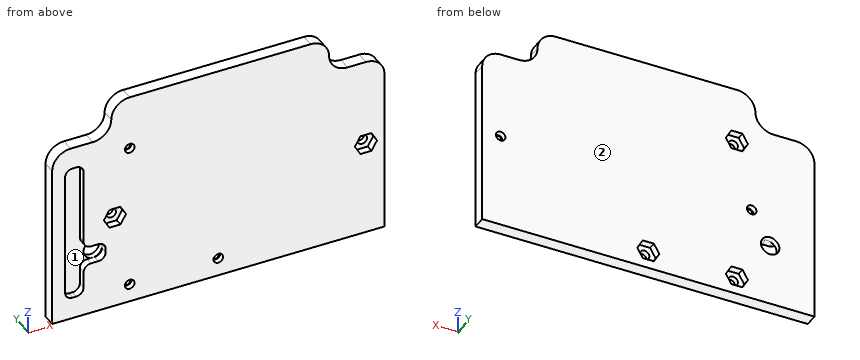
```python
from build123d import *

# Parameters (mm, degrees)
F1_DEPTH  = 4.445
F2_R      = 1.651
F3_DEPTH  = 4.446
F4_R      = 1.651
F5_DEPTH  = 4.446
F7_DEPTH  = 2.54
F9_DEPTH  = 2.54
F10_R     = 3.175
F11_DEPTH = 4.446
F13_DEPTH = 2.54


with BuildPart() as f1:
    # F0 (on Front) → F1 (new body)
    with BuildSketch(Plane.XZ):
        with BuildLine():
            Line((33.804538, 40.817322), (-28.425462, 40.817322))
            ThreePointArc((-28.425462, 40.817322), (-32.91559, 38.95745), (-34.775462, 34.467322))
            ThreePointArc((-34.775462, 34.467322), (-36.635334, 29.977194), (-41.125462, 28.117322))
            Line((-41.125462, 28.117322), (-48.745462, 28.117322))
            ThreePointArc((-48.745462, 28.117322), (-53.23559, 26.25745), (-55.095462, 21.767322))
            Line((-55.095462, 21.767322), (-55.095462, -35.382678))
            Line((-55.095462, -35.382678), (59.204538, -35.382678))
            Line((59.204538, -35.382678), (59.204538, 21.767322))
            ThreePointArc((59.204538, 21.767322), (57.344666, 26.25745), (52.854538, 28.117322))
            Line((52.854538, 28.117322), (46.504538, 28.117322))
            ThreePointArc((46.504538, 28.117322), (42.01441, 29.977194), (40.154538, 34.467322))
            ThreePointArc((40.154538, 34.467322), (38.294666, 38.95745), (33.804538, 40.817322))
        make_face()
    extrude(amount=F1_DEPTH)

    # F2 (on face) → F3 (cut, through all)
    with BuildSketch(Plane.XZ.offset(4.445)):
        with Locations((-28.425462, -29.032678)):
            Circle(F2_R)
        with Locations((2.054538, -29.032678)):
            Circle(F2_R)
        with Locations((-28.425462, 21.767322)):
            Circle(F2_R)
    extrude(amount=-F3_DEPTH, mode=Mode.SUBTRACT)

    # F4 (on face) → F5 (cut, through all)
    with BuildSketch(Plane.XZ.offset(4.445)):
        with Locations((-33.505462, -2.362678)):
            Circle(F4_R)
        with Locations((52.854538, -2.362678)):
            Circle(F4_R)
    extrude(amount=-F5_DEPTH, mode=Mode.SUBTRACT)

    # F6 (on face) → F7 (cut)
    with BuildSketch(Plane.XZ.offset(4.445)):
        Polygon((-29.695462, -2.362678), (-31.600462, 0.936879), (-35.410462, 0.936879), (-37.315462, -2.362678), (-35.410462, -5.662235), (-31.600462, -5.662235), align=None)
        Polygon((54.759538, 0.936879), (50.949538, 0.936879), (49.044538, -2.362678), (50.949538, -5.662235), (54.759538, -5.662235), (56.664538, -2.362678), align=None)
    extrude(amount=-F7_DEPTH, mode=Mode.SUBTRACT)

    # F8 (on face) → F9 (cut)
    with BuildSketch(Plane(origin=(0, 0, 0), x_dir=(-1, 0, 0), z_dir=(0, 1, 0))):
        Polygon((30.330462, 18.467765), (32.235462, 21.767322), (30.330462, 25.066879), (26.520462, 25.066879), (24.615462, 21.767322), (26.520462, 18.467765), align=None)
        Polygon((32.235462, -29.032678), (30.330462, -25.733121), (26.520462, -25.733121), (24.615462, -29.032678), (26.520462, -32.332235), (30.330462, -32.332235), align=None)
        Polygon((-0.149538, -25.733121), (-3.959538, -25.733121), (-5.864538, -29.032678), (-3.959538, -32.332235), (-0.149538, -32.332235), (1.755462, -29.032678), align=None)
    extrude(amount=-F9_DEPTH, mode=Mode.SUBTRACT)

    # F10 (on face) → F11 (cut, through all)
    with BuildSketch(Plane(origin=(0, 0, 0), x_dir=(-1, 0, 0), z_dir=(0, 1, 0))):
        with Locations((39.855462, -13.792678)):
            Circle(F10_R)
    extrude(amount=-F11_DEPTH, mode=Mode.SUBTRACT)

    # F12 (on face) → F13 (cut)
    with BuildSketch(Plane.XZ.offset(4.445)):
        with BuildLine():
            Line((-46.840462, 20.497322), (-48.110462, 20.497322))
            ThreePointArc((-48.110462, 20.497322), (-49.906513, 19.753373), (-50.650462, 17.957322))
            Line((-50.650462, 17.957322), (-50.650462, -10.617678))
            Line((-50.650462, -10.617678), (-50.650462, -16.967678))
            Line((-50.650462, -16.967678), (-50.650462, -25.222678))
            ThreePointArc((-50.650462, -25.222678), (-49.906513, -27.018729), (-48.110462, -27.762678))
            Line((-48.110462, -27.762678), (-46.840462, -27.762678))
            ThreePointArc((-46.840462, -27.762678), (-45.044411, -27.018729), (-44.300462, -25.222678))
            Line((-44.300462, -25.222678), (-44.300462, -19.507678))
            ThreePointArc((-44.300462, -19.507678), (-43.556513, -17.711627), (-41.760462, -16.967678))
            Line((-41.760462, -16.967678), (-39.220462, -16.967678))
            ThreePointArc((-39.220462, -16.967678), (-37.424411, -16.223729), (-36.680462, -14.427678))
            Line((-36.680462, -14.427678), (-36.680462, -13.157678))
            ThreePointArc((-36.680462, -13.157678), (-37.424411, -11.361627), (-39.220462, -10.617678))
            Line((-39.220462, -10.617678), (-41.760462, -10.617678))
            ThreePointArc((-41.760462, -10.617678), (-43.556513, -9.873729), (-44.300462, -8.077678))
            Line((-44.300462, -8.077678), (-44.300462, 17.957322))
            ThreePointArc((-44.300462, 17.957322), (-45.044411, 19.753373), (-46.840462, 20.497322))
        make_face()
    extrude(amount=-F13_DEPTH, mode=Mode.SUBTRACT)


solid = f1.part
```
CAD build for the part. Positions are in the model's coordinates, mm. Face numbers are marked on the shaded views. Round coordinates to 2 decimals unless told otherwise and drop trailing zeros. Order: outer loops, then holes, each group sorted by start corner. A loop starts at its lowest first (then second) coordinate and runs counter-clockwise, first axis right, second up. Notation, with made-up numbers: (-35.5, 30) - (-9.5, 30) arc R5 cw to (-9.5, 39) - close; hole circle Ø4 at (45.25, 37.5). An arc over 180 degrees is marked (long way). Use CSV: the item, a comma, the result in double quotes. Start each with the question number.
1) Saw through at A-A (y = -1.1). Count the separate pieces of the cut face and the enclosed holes in it, and give its area (3 significant figures).
2) Pin check, flat tips, straight feed: pin 1 Ø1 at (x, y) = (-47.5, -3.5) entering from +Z; pin 2 Ø7.5 at (x, z) = (-29, 20) entering from +Y; pin 3 Ø2 at (x, z) = (-27, -29.5) entering from +Y; pin 4 Ø0.8 at (x, y) = (-29, -1) entering from +Z. Stop position of each tip, or through.
3) Saw through at D-D (z = 36). List the corners of the cut face in (x, y) (3 decimals), and give its area (3 significant figures).
4) Two-plate mould, pull along Z, no slides. Class the marked faces 1 and 2: pulls with the +Z half, pulls with the -Z half, needs draft (parallel to the pull), parting line crosses it, or undercut.
5) Wall check: L1, parallel to Z at x = -29, y = -2; L2, parallel to X at y = -1.3, z = -31; L3, parallel to X at y = -2.9, z = -24.5. Give the ranges that are in metal, low to high. Write a range as [from, to].
6) Saw through at B-B (z = -23). List the corners of the cut face in (x, y) (3 decimals), and give its area (3 significant figures).
7) Saw through at C-C (x = 44). List the corners of the cut face in (y, z) (3 decimals).
Values follow:
1,separate pieces,"1"
1,enclosed holes,"6"
1,area,"8,030 mm2"
2,pin 1,"stops at z = 28.12"
2,pin 2,"stops at y = 0"
2,pin 3,"stops at y = -2.54"
2,pin 4,"stops at z = 40.81"
3,outline,"(-34.588, -4.445) - (39.967, -4.445) - (39.967, 0) - (-34.588, 0) - close"
3,area,"331 mm2"
4,face 1,"undercut"
4,face 2,"needs draft"
5,L1,"z = [-35.38, -32.33], [-25.73, 18.47], [25.07, 40.79]"
5,L2,"x = [-55.1, -31.1], [-25.75, -0.62], [4.73, 59.2]"
5,L3,"x = [-55.1, -50.65], [-44.3, 59.2]"
6,outline,"(-55.095, -4.445) - (-50.65, -4.445) - (-50.65, -1.905) - (-44.3, -1.905) - (-44.3, -4.445) - (59.205, -4.445) - (59.205, 0) - (-55.095, 0) - close"
6,area,"492 mm2"
7,outline,"(-4.445, -35.383) - (0, -35.383) - (0, 28.632) - (-4.445, 28.632) - close"
